Input: part model. Units: mm. Frame: model coordinates. Coordinates: 2 decimals unless noted, no trailing zeros. Loops run counter-clockwise (first coordinate to the right, second up) from the corner with the lowest first, then second, coordinate; pieces in that order, holes last. Notation, with made-up numbers: (54, 46) -> (86, 46) arc R3 ccw to (86, 50) -> close; hole circle Ø1 at (88.25, 15). An arc over 180 degrees is marked (long way). Put each result on its own line as item: value. Start each with the question number.
1) Contact query for flat-ended pins moving along their axis: P1, Ø5.5, axis at x = 0, z = 25.4, coming from the +Y side; P2, Ø1, axis at y = -11, z = 24.5, coming from the +X side. Output: stop coordinate, or through.
2) Cut plane A-A (z = -25.4). Return the cut outline in (x, y) (3 decimals).
3) Cut plane D-D (z = 40.5). Return the cut outline in (x, y), plus the area to 3 significant figures.
4) Material intervals for L1, parallel to Z at x = 0, y = -3.5 (3 decimals); L2, parallel to Z at x = 0, y = -8; L3, parallel to Y at x = -5, z = 26.5, sorted ascending.
5) Cut plane B-B (x = 0). Return the cut outline in (y, z) (3 decimals).
6) Cut plane C-C (y = -9.25). Return the cut outline in (x, z), plus the area to 3 significant figures.
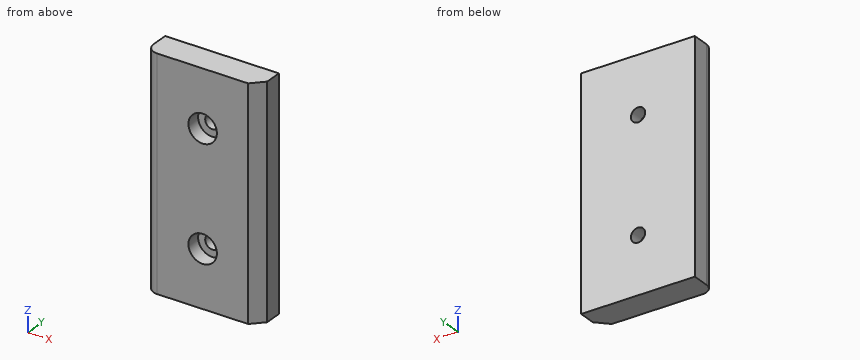
from build123d import *

# Parameters (mm, degrees)
F0_W           = 50.8
F0_H           = 101.6
F1_DEPTH       = 12.7
F3_D           = 6.35
F3_CBORE_D     = 12.7
F3_CBORE_DEPTH = 6.35
F4_R           = 5.08
F5_SIZE        = 5.08


with BuildPart() as f1:
    # F0 (on Front) → F1 (new body)
    with BuildSketch(Plane.XZ):
        Rectangle(F0_W, F0_H)
    extrude(amount=F1_DEPTH)

    # F3 (through all)
    with Locations(Plane.XZ.offset(12.7)):
        with Locations((0, 25.4), (0, -25.4)):
            CounterBoreHole(F3_D / 2, F3_CBORE_D / 2, F3_CBORE_DEPTH)

    # F4
    f4_edges = [f1.edges().sort_by_distance(p)[0] for p in [
        (-25.4, -12.7, 0),
    ]]
    fillet(f4_edges, radius=F4_R)

    # F5
    f5_edges = [f1.edges().sort_by_distance(p)[0] for p in [
        (25.4, -12.7, 0),
    ]]
    chamfer(f5_edges, length=F5_SIZE)


solid = f1.part
Results found:
1. P1: passes through
1. P2: stops at x = 22.52
2. outline: (-25.4, -7.62) arc R5.08 ccw to (-20.32, -12.7) -> (-6.35, -12.7) -> (-6.35, -6.35) -> (-3.175, -6.35) -> (-3.175, 0) -> (-25.4, 0) -> close; (3.175, -6.35) -> (6.35, -6.35) -> (6.35, -12.7) -> (20.32, -12.7) -> (25.4, -7.62) -> (25.4, 0) -> (3.175, 0) -> close
3. outline: (-25.4, -7.62) arc R5.08 ccw to (-20.32, -12.7) -> (20.32, -12.7) -> (25.4, -7.62) -> (25.4, 0) -> (-25.4, 0) -> close
3. area: 627 mm2
4. L1: z = -50.8 to -28.575, -22.225 to 22.225, 28.575 to 50.8
4. L2: z = -50.8 to -31.75, -19.05 to 19.05, 31.75 to 50.8
4. L3: y = -6.35 to 0
5. outline: (-12.7, -50.8) -> (0, -50.8) -> (0, -28.575) -> (-6.35, -28.575) -> (-6.35, -31.75) -> (-12.7, -31.75) -> close; (-12.7, -19.05) -> (-6.35, -19.05) -> (-6.35, -22.225) -> (0, -22.225) -> (0, 22.225) -> (-6.35, 22.225) -> (-6.35, 19.05) -> (-12.7, 19.05) -> close; (-12.7, 31.75) -> (-6.35, 31.75) -> (-6.35, 28.575) -> (0, 28.575) -> (0, 50.8) -> (-12.7, 50.8) -> close
6. outline: (-25.13, -50.8) -> (23.77, -50.8) -> (23.77, 50.8) -> (-25.13, 50.8) -> close; hole circle Ø12.7 at (0, -25.4); hole circle Ø12.7 at (0, 25.4)
6. area: 4,720 mm2
